Could you check a few things on this model? Use its own coordinates, in mm. A direction names the side the tool comes from. Give positions to 0.01 mm unless a question says otherwise; leave off trailing zeros. Write each loop counter-clockwise with the first axis right and the second up, starting at its lowest first coordinate (ties: lowest second). Pieces come first, ordered by that corner, then holes. Notation, with made-up numbers: (41.25, 63.5) - (54.25, 63.5) arc R20 ccw to (54.25, 81.5) - close; hole circle Ø11 at (-12, 86.5). An arc over 180 degrees is marked (long way). Answer in a Markdown table with one row per item.
from build123d import *

# Parameters (mm, degrees)
RESSALTO_EXTRUS_O1_DEPTH = 30


with BuildPart() as part:
    # Esboço1 → Revolução1 (revolve)
    with BuildSketch(Plane.XY):
        with BuildLine():
            Line((0, 40), (10, 30))
            Line((10, 30), (125, 30))
            ThreePointArc((125, 30), (128.535533906, 31.464466094), (130, 35))
            Line((130, 35), (130, 40))
            Line((130, 40), (150, 40))
            Line((150, 40), (150, 50))
            Line((150, 50), (120, 50))
            Line((120, 50), (120, 75))
            Line((120, 75), (110, 75))
            Line((110, 75), (110, 50))
            ThreePointArc((110, 50), (107.071067812, 42.928932188), (100, 40))
            Line((100, 40), (30, 40))
            Line((30, 40), (20, 50))
            Line((20, 50), (0, 50))
            Line((0, 50), (0, 40))
        make_face()
    revolve(axis=Axis((0, 0, 0), (1, 0, 0)))

    # Esboço2 → Ressalto-extrusão1 (add)
    with BuildSketch(Plane(origin=(150, 0, 0), x_dir=(0, 0, -1), z_dir=(1, 0, 0))):
        with BuildLine():
            Line((-50, 50), (-50, 2.4e-08))
            ThreePointArc((-50, 2.4e-08), (-35.355339059, 35.35533906), (-2.3e-08, 50))
            Line((-2.3e-08, 50), (-50, 50))
        make_face()
        with BuildLine():
            Line((-50, 2.4e-08), (-50, -50))
            Line((-50, -50), (2.3e-08, -50))
            ThreePointArc((2.3e-08, -50), (-35.35533906, -35.355339059), (-50, 2.4e-08))
        make_face()
        with BuildLine():
            ThreePointArc((50, 0), (35.355339067, -35.355339051), (2.3e-08, -50))
            Line((2.3e-08, -50), (50, -50))
            Line((50, -50), (50, 0))
        make_face()
        with BuildLine():
            ThreePointArc((-2.3e-08, 50), (35.355339051, 35.355339067), (50, 0))
            Line((50, 0), (50, 50))
            Line((50, 50), (-2.3e-08, 50))
        make_face()
    extrude(amount=-RESSALTO_EXTRUS_O1_DEPTH)


solid = part.part
1) Will these pins go through, and if not, where does the flat tip stop? P1, Ø8, axis at x = 35.5, z = -13.5, coming from the -Y side; P2, Ø12, axis at x = 75.5, z = 22, coming from the -Y side; P3, Ø24, axis at x = 142.5, z = 23.5, coming from the +Y side.
Check values:
| item | result |
|---|---|
| P1 | stops at y = -38.86 |
| P2 | stops at y = -36.66 |
| P3 | stops at y = 50 |
2) Imagine slicing it at C-C (x = 23.5). List the corners of the cut face in (y, z) for me.
Check values:
| item | result |
|---|---|
| outline | circle Ø93 at (0, 0); hole circle Ø60 at (0, 0) |
3) Imagine slicing it at D-D (z = 53.5). List the corners of the cut face in (x, y) for me, then the cut area to 3 significant figures.
Check values:
| item | result |
|---|---|
| outline | (110, -52.56) - (120, -52.56) - (120, 52.56) - (110, 52.56) - close |
| area | 1,050 mm2 |
4) We'd pull the mould along Z, two halves only. Please class faces 1 (the face through (68.31, -29.97, 1.32)), 2 (the face through (29, -9, -40)), 3 (the face through (110, 49, -16)): +Z half, -Z half, draft (parallel to the pull), parting line (faces both ways), or undercut.
Check values:
| item | result |
|---|---|
| face 1 | undercut |
| face 2 | parting line |
| face 3 | draft |
5) If I drill on line 1 (Z direction, x = 85, y = 0); line 2 (Z direction, x = 143.25, y = 0); line 3 (X direction, y = 55.5, z = 12), over which ranges is the centre line in solid material (lowest first)?
Check values:
| item | result |
|---|---|
| line 1 | z = -40 to -30, 30 to 40 |
| line 2 | z = -50 to -40, 40 to 50 |
| line 3 | x = 110 to 120 |
6) On a 3-axis mill with a long thin cutter (end or side, diameter ignored), from which of +Z, -Z, +X, -X, +Y, -Y can I reach the whole of each face in a straight line? I mean faces 4 (the face through (135, -1, -50)), 5 (the face through (135, 50, -1)), 6 (the face through (9.86, 47.69, 15.02)), 7 (the face through (64.51, -8.67, -39.05)). Say none if no direction works.
Check values:
| item | result |
|---|---|
| face 4 | -Z, +X, +Y, -Y |
| face 5 | +Z, -Z, +X, +Y |
| face 6 | -X |
| face 7 | none |
